Source: CAD feature listing. Evaluate the final solid. Frame: model axes, mm. A direction names the side the tool comes from. Round coordinates to 2 decimals unless told otherwise and drop trailing zeros. Use one line per item in the form item = value. Start each with the question number.
Q1. Pin query (flat end, axial travel): pin 1 Ø17 at (x, y) = (18.5, 11.5) entering from +Z; pin 2 Ø1.5 at (x, y) = (-5.5, 17.5) entering from -Z; pin 3 Ø23.5 at (x, y) = (-10.5, 14) entering from +Z. Return the tip coordinate at first contact, or that it passes through.
Q2. Ray query, line 1 (Z direction, x = 14, y = 16); line 2 (Z direction, x = -6.5, y = -13.5); line 3 (X direction, y = -20.5, z = 2.5). Return the intervals inside material, ascending. Write a range as [from, to].
Q3. Set-up query: faces 1 (the flat face through (-20, 19, 0)), 2 (the flat face through (20, 19, 0)), 3 (the flat face through (20, -19, 0)), 4 (the flat face through (-20, -19, 0)). Return all of +Z, -Z, +X, -X, +Y, -Y with unobstructed straight access to the full face (end or side cutting, diameter ignored); none if empty.
from build123d import *

# Parameters (mm, degrees)
F0_R     = 25
F1_DEPTH = 10
F4_DEPTH = 25
F5_DEPTH = 25


# Not quite as in the source:
# - a fillet or chamfer that OpenCascade refuses, or shapes differently, is made with other operations: its cross-section is extruded or revolved along the edge and cut away or added


with BuildPart() as f1:
    # F0 (on Top) → F1 (new body)
    with BuildSketch(Plane.XY):
        Circle(F0_R)
    extrude(amount=F1_DEPTH)

    # F2: fillet of radius 25 on 1 edges, made by hand

    # F2_s1 → F2_t2 (revolve, cut)
    with BuildSketch(Plane.XZ):
        with BuildLine():
            ThreePointArc((25, 0), (16.1803398875, 7.360679775), (5, 10))
            Line((5, 10), (25, 10))
            Line((25, 10), (25, 0))
        make_face()
    revolve(axis=Axis((0, 0, 10), (0, 0, 1)), mode=Mode.SUBTRACT)

    # F3 (on Right) → F4 (join)
    with BuildSketch(Plane.YZ):
        with BuildLine():
            add(Edge.make_bspline(
                [(24.730604142, 0), (17.4811016216, -6.4583238577), (3.1217539474, -19.2505557941), (1.033815633, -37.8348617707), (0, -47.0366403461)],
                knots=[0, 0, 0, 0, 0.5048629426, 1, 1, 1, 1], degree=3))
            Line((24.730604142, 0), (-24.730604142, 0))
            add(Edge.make_bspline(
                [(-24.730604142, 0), (-17.4811016216, -6.4583238577), (-3.1217539474, -19.2505557941), (-1.033815633, -37.8348617707), (0, -47.0366403461)],
                knots=[0, 0, 0, 0, 0.5048629426, 1, 1, 1, 1], degree=3))
        make_face()
    extrude(amount=F4_DEPTH)

    # F5 (add): a face of the model
    f5_faces = [f1.faces().sort_by_distance(p)[0] for p in [
        (0, 0, -11.4252371801),
    ]]
    extrude(f5_faces, amount=F5_DEPTH)


solid = f1.part
Completed:
q1.pin_1 = 8.59
q1.pin_2 = -7.33
q1.pin_3 = 9.99
q2.line_1 = [-8.07, 3.99]
q2.line_2 = [-10.67, 7.92]
q2.line_3 = [-10.1, 10.1]
q3.face_1 = +Z, -X, +Y
q3.face_2 = +Z, +X, +Y
q3.face_3 = +Z, +X, -Y
q3.face_4 = +Z, -X, -Y
